from build123d import *

# Parameters (mm, degrees)
F1_DEPTH = 6.35
F0_W     = 298.45
F0_H     = 288.925
F2_DEPTH = 12.7
F3_W     = 50.8
F3_H     = 6.35
F4_DEPTH = 295.276


with BuildPart() as f1:
    # F0 (on Top) → F1 (new body)
    with BuildSketch(Plane.XY):
        Polygon((0, 295.275), (0, 0), (6.35, 0), (6.35, 288.925), (304.8, 288.925), (304.8, 0), (311.15, 0), (311.15, 295.275), align=None)
    extrude(amount=F1_DEPTH)

    # F0 (on Top) → F2 (join)
    with BuildSketch(Plane.XY):
        with Locations((155.575, 144.4625)):
            Rectangle(F0_W, F0_H)
    extrude(amount=F2_DEPTH)

    # F3 (on face) → F4 (cut, through all)
    with BuildSketch(Plane.XZ):
        with Locations((155.575, 9.525)):
            Rectangle(F3_W, F3_H)
    extrude(amount=-F4_DEPTH, mode=Mode.SUBTRACT)


solid = f1.part
Geometry: final body of the model. Coordinates: model frame, mm. Give positions to 0.01 mm unless a question says otherwise; leave off trailing zeros. Order: outer loops, then holes, each group sorted by start corner. A loop starts at its lowest first (then second) coordinate and runs counter-clockwise, first axis right, second up. Notation, with made-up numbers: (7, -20.5) -> (38, -20.5) arc R27 cw to (38, -1.5) -> close; hole circle Ø1 at (-33.75, 22). An arc over 180 degrees is marked (long way). Answer as a JSON object with one key per item and string values.
Q1. Section A-A (z = 8.5). Output: boundary loops of the cut face in (x, y) (3 decimals), plus the area to 3 significant figures.
Entries:
{"outline": "(6.35, 0) -> (130.175, 0) -> (130.175, 288.925) -> (6.35, 288.925) -> close; (180.975, 0) -> (304.8, 0) -> (304.8, 288.925) -> (180.975, 288.925) -> close", "area": "71,600 mm^2"}
Q2. Material intervals for probe 1 along X at (y, z) = (185, 10.25) (3 decimals); probe 2 along Y at (x, z) = (243, 11.75) (3 decimals), sorted ascending.
Entries:
{"probe 1": "x = 6.35 to 130.175, 180.975 to 304.8", "probe 2": "y = 0 to 288.925"}
Q3. First-contact query: pin 1 (5 mm diameter, centred on x = 235, z = 10.5, fed in from +Y) (3 decimals); pin 2 (7 mm diameter, centred on y = 213.5, z = 10.5, fed in from +X); pin 3 (3 mm diameter, centred on y = 79, z = 10.5, fed in from -X). Flat tips, straight axial feed; report the tip coordinate or a pass-through.
Entries:
{"pin 1": "stops at y = 288.925", "pin 2": "stops at x = 304.8", "pin 3": "stops at x = 6.35"}
Q4. Section C-C (x = 150). Output: boundary loops of the cut face in (y, z) (3 decimals).
Entries:
{"outline": "(0, 0) -> (295.275, 0) -> (295.275, 6.35) -> (0, 6.35) -> close"}
Q5. Draft query along X for faces 1 (the flat face through (67, 146, 12.7)), 2 (the flat face through (132, 159, 6.35)). Return one class per face: released by +X, released by -X, zero draft, split by the parting line, or undercut.
Entries:
{"face 1": "zero draft", "face 2": "undercut"}
Q6. Section B-B (y = 250.5). Output: boundary loops of the cut face in (x, z) (3 decimals).
Entries:
{"outline": "(0, 0) -> (311.15, 0) -> (311.15, 6.35) -> (304.8, 6.35) -> (304.8, 12.7) -> (180.975, 12.7) -> (180.975, 6.35) -> (130.175, 6.35) -> (130.175, 12.7) -> (6.35, 12.7) -> (6.35, 6.35) -> (0, 6.35) -> close"}
